Read the model definition and answer for the solid it produces. Units are mm, in the model's axes. Face numbers are marked on the shaded views. A direction names the side the tool comes from. Give positions to 0.01 mm unless a question says otherwise; leave off trailing zeros. Loops run counter-clockwise (first coordinate to the right, second up) from the corner with the lowest first, then second, coordinate; pieces in that order, holes last.
(1) Find section C-C, the plane z = 0. Write down the section's boundary in (x, y).
(2) Find section B-B, the plane x = 0.95. Write down the section's boundary in (y, z).
(3) Which of the six approach directions +Z, -Z, +X, -X, +Y, -Y give full straight-line access (tool end or side, diameter ignored) to the marked faces 1 and 2?
(4) Straight lines are drawn through the part: probe 1 along Y at (x, z) = (0.55, 0.3); probe 2 along Y at (x, z) = (-0.15, 1.1); probe 3 along X at (y, z) = (6.5, 0.05). For each, find the intervals that lie inside material, in ascending order.
(5) Each of these flat-tipped pins is pushed along its axis until it touches: P1, Ø1, axis at y = 1, z = -0.5, coming from the +X side; P2, Ø0.6, axis at x = 0, y = 8, coming from the -Z side; P3, Ø1.4, axis at x = 1, z = 0, coming from the -Y side; P4, Ø1, axis at x = -1.5, y = 6, coming from the -Z side. Where does it stop, or does it pass through?
(6) Find section A-A, the plane z = -0.75. Write down the section's boundary in (x, y).
(7) Find section D-D, the plane y = 5. Write down the section's boundary in (x, z).
```python
from build123d import *

# Parameters (mm, degrees)
SKETCH_1_R          = 2.5
EXTRUDE_1_DEPTH     = 3
SKETCH_2_R          = 0.187953655
EXTRUDE_2_DEPTH     = 7.3
CUT_EXTRUDE_START   = -2.3
SKETCH_4_R          = 0.187953655
CUT_EXTRUDE_1_DEPTH = 2.3
SKETCH_6_R          = 2.392138428
EXTRUDE_3_DEPTH     = 4.7
SKETCH_7_W          = 0.880091412
SKETCH_7_H          = 4.366078492
CUT_EXTRUDE_3_DEPTH = 0.5
EXTRUDE_4_DEPTH     = 1
EXTRUDE_5_DEPTH     = 4
SKETCH_11_W         = 0.290967458
SKETCH_11_H         = 0.085529097
CUT_EXTRUDE_4_DEPTH = 1


with BuildPart() as part:
    # 草图1 → 凸台-拉伸1 (new body)
    with BuildSketch(Plane(origin=(0, 0, 0), x_dir=(1, 0, 0), z_dir=(0, 1, 0))):
        with Locations(Location((0, 0, 0), (0, 0, 270))):
            Circle(SKETCH_1_R)
    extrude(amount=EXTRUDE_1_DEPTH)

    # 草图2 → 凸台-拉伸2 (add)
    with BuildSketch(Plane(origin=(0, 3, 0), x_dir=(1, 0, 0), z_dir=(0, 1, 0))):
        with Locations(Location((0, 0, 0), (0, 0, 270))):
            Circle(SKETCH_2_R)
    extrude(amount=EXTRUDE_2_DEPTH)

    # 草图4 → 切除-拉伸1 (cut)
    with BuildSketch(Plane(origin=(0, 10.3, 0), x_dir=(1, 0, 0), z_dir=(0, 1, 0)).offset(CUT_EXTRUDE_START)):
        with Locations(Location((0, 0, 0), (0, 0, 270))):
            Circle(SKETCH_4_R)
    extrude(amount=CUT_EXTRUDE_1_DEPTH, mode=Mode.SUBTRACT)

    # 草图6 → 凸台-拉伸3 (add)
    with BuildSketch(Plane(origin=(0, 8, 0), x_dir=(1, 0, 0), z_dir=(0, 1, 0))):
        with Locations(Location((0, 0, 0), (0, 0, 270))):
            Circle(SKETCH_6_R)
    extrude(amount=-EXTRUDE_3_DEPTH)

    # 草图7 → 切除-拉伸3 (cut)
    with BuildSketch(Plane(origin=(0, 8, 0), x_dir=(1, 0, 0), z_dir=(0, 1, 0))):
        Rectangle(SKETCH_7_W, SKETCH_7_H)
    extrude(amount=-CUT_EXTRUDE_3_DEPTH, mode=Mode.SUBTRACT)

    # 草图9 → 凸台-拉伸4 (add)
    with BuildSketch(Plane.XZ):
        Polygon((0, 2.448076853), (0.473512734, 2.454747582), (0.473512734, 2.362547756), (-0.506872491, 2.362547756), (-0.506872491, 2.448076853), align=None)
    extrude(amount=EXTRUDE_4_DEPTH)

    # 草图10 → 凸台-拉伸5 (add)
    with BuildSketch(Plane(origin=(0, 3, 0), x_dir=(1, 0, 0), z_dir=(0, 1, 0))):
        Polygon((-1.457651402, 1.928637822), (-1.767058539, 1.928637822), (-1.767058539, 2.038649249), (-1.447034637, 2.038649249), align=None)
        Polygon((1.478278545, 1.928637822), (1.447034637, 2.038649249), (1.794561396, 2.038649249), (1.794561396, 1.928637822), align=None)
    extrude(amount=-EXTRUDE_5_DEPTH)

    # 草图11 → 切除-拉伸4 (cut)
    with BuildSketch(Plane.XZ.offset(1)):
        with Locations((-0.361388762, 2.405312305)):
            Rectangle(SKETCH_11_W, SKETCH_11_H)
        Polygon((0.105106814, 2.449557571), (0.105106814, 2.362547756), (0.473512734, 2.362547756), (0.473512734, 2.454747582), align=None)
    extrude(amount=-CUT_EXTRUDE_4_DEPTH, mode=Mode.SUBTRACT)


solid = part.part
```
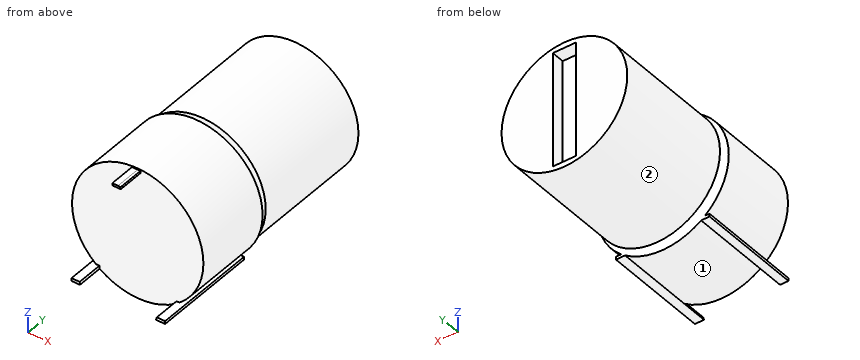
Entries:
1. outline: (-2.5, 0) - (2.5, 0) - (2.5, 3) - (0.19, 3) - (0.19, 3.3) - (2.39, 3.3) - (2.39, 8) - (0.44, 8) - (0.44, 7.5) - (-0.44, 7.5) - (-0.44, 8) - (-2.39, 8) - (-2.39, 3.3) - (-0.19, 3.3) - (-0.19, 3) - (-2.5, 3) - close
2. outline: (0, -2.31) - (3, -2.31) - (3, 2.31) - (0, 2.31) - close; (3.3, -2.2) - (8, -2.2) - (8, 2.2) - (3.3, 2.2) - close
3. face 1: -Z, +Y, -Y
3. face 2: +Y
4. probe 1: y = 0 to 3, 3.3 to 8
4. probe 2: y = 0 to 3, 3.3 to 7.5
4. probe 3: x = -2.39 to 2.39
5. P1: stops at x = 2.5
5. P2: stops at z = -2.39
5. P3: stops at y = 0
5. P4: stops at z = -2.17
6. outline: (-2.38, 0) - (2.38, 0) - (2.38, 3) - (-2.38, 3) - close; (-2.27, 3.3) - (2.27, 3.3) - (2.27, 8) - (0.44, 8) - (0.44, 7.5) - (-0.44, 7.5) - (-0.44, 8) - (-2.27, 8) - close
7. outline: circle Ø4.78 at (0, 0)
